from build123d import *

# Parameters (mm, degrees)
SKETCH1_W                           = 96.1517
SKETCH1_H                           = 78.74
BASE_PLATE_DEPTH                    = 2
SKETCH2_W                           = 5.08
SKETCH2_H                           = 5.08
SERVO_SUPPORTS_DEPTH                = 27.94
SKETCH3_R                           = 0.635
SERVO_MOUNT_HOLES_DEPTH             = 12.7
STRAP_HOLES_REACH                   = 70.132
SERVO_MOUNT_SPACING_COUNT           = 2
SERVO_MOUNT_SPACING_PITCH           = 38.1
SERVO_MOUNT_SPACING_COPY_1_SKETCH_W = 5.08
SERVO_MOUNT_SPACING_COPY_1_SKETCH_H = 5.08
SERVO_MOUNT_SPACING_COPY_1_DEPTH    = 27.94
SERVO_MOUNT_SPACING_COPY_2_SKETCH_R = 0.635
SERVO_MOUNT_SPACING_COPY_2_DEPTH    = 12.7
SKETCH11_W                          = 2.54
SKETCH11_H                          = 39.37
RACK_RAILS_DEPTH                    = 2.54


with BuildPart() as part:
    # Sketch1 → Base Plate (new body)
    with BuildSketch(Plane(origin=(0, 0, 0), x_dir=(1, 0, 0), z_dir=(0, 1, 0))):
        Rectangle(SKETCH1_W, SKETCH1_H)
    extrude(amount=BASE_PLATE_DEPTH)

    # Sketch2 → Servo Supports (add)
    with BuildSketch(Plane(origin=(0, 2, 0), x_dir=(1, 0, 0), z_dir=(0, 1, 0))):
        with Locations((20.13585, -30.48)):
            Rectangle(SKETCH2_W, SKETCH2_H)
        with Locations((20.13585, -2.54)):
            Rectangle(SKETCH2_W, SKETCH2_H)
    servo_supports = extrude(amount=SERVO_SUPPORTS_DEPTH)

    # Sketch3 → Servo Mount Holes (cut)
    with BuildSketch(Plane(origin=(22.67585, 0, 0), x_dir=(0, 0, -1), z_dir=(1, 0, 0))):
        with Locations((-30.504257117, 23.59)):
            Circle(SKETCH3_R)
        with Locations((-2.792857117, 23.59)):
            Circle(SKETCH3_R)
    servo_mount_holes = extrude(amount=-SERVO_MOUNT_HOLES_DEPTH, mode=Mode.SUBTRACT)

    # Sketch4 → Strap Holes (cut, up to next)
    with BuildSketch(Plane(origin=(0, 2, 0), x_dir=(1, 0, 0), z_dir=(0, 1, 0)), mode=Mode.PRIVATE) as strap_holes_sk1:
        with BuildLine():
            Line((45.53585, -24.17), (45.53585, -33.02))
            ThreePointArc((45.53585, -33.02), (44.53585, -34.02), (43.53585, -33.02))
            Line((43.53585, -33.02), (43.53585, -24.17))
            ThreePointArc((43.53585, -24.17), (44.53585, -23.17), (45.53585, -24.17))
        make_face()
    strap_holes_tool1 = extrude(strap_holes_sk1.sketch, amount=-STRAP_HOLES_REACH, mode=Mode.PRIVATE) & part.part
    # Sketch4 → Strap Holes (cut, up to next)
    with BuildSketch(Plane(origin=(0, 2, 0), x_dir=(1, 0, 0), z_dir=(0, 1, 0)), mode=Mode.PRIVATE) as strap_holes_sk2:
        with BuildLine():
            Line((45.53585, 33.02), (45.53585, 24.17))
            ThreePointArc((45.53585, 24.17), (44.53585, 23.17), (43.53585, 24.17))
            Line((43.53585, 24.17), (43.53585, 33.02))
            ThreePointArc((43.53585, 33.02), (44.53585, 34.02), (45.53585, 33.02))
        make_face()
    strap_holes_tool2 = extrude(strap_holes_sk2.sketch, amount=-STRAP_HOLES_REACH, mode=Mode.PRIVATE) & part.part
    # Sketch4 → Strap Holes (cut, up to next)
    with BuildSketch(Plane(origin=(0, 2, 0), x_dir=(1, 0, 0), z_dir=(0, 1, 0)), mode=Mode.PRIVATE) as strap_holes_sk3:
        with BuildLine():
            Line((-43.63085, -24.17), (-43.63085, -33.02))
            ThreePointArc((-43.63085, -33.02), (-44.63085, -34.02), (-45.63085, -33.02))
            Line((-45.63085, -33.02), (-45.63085, -24.17))
            ThreePointArc((-45.63085, -24.17), (-44.63085, -23.17), (-43.63085, -24.17))
        make_face()
    strap_holes_tool3 = extrude(strap_holes_sk3.sketch, amount=-STRAP_HOLES_REACH, mode=Mode.PRIVATE) & part.part
    # Sketch4 → Strap Holes (cut, up to next)
    with BuildSketch(Plane(origin=(0, 2, 0), x_dir=(1, 0, 0), z_dir=(0, 1, 0)), mode=Mode.PRIVATE) as strap_holes_sk4:
        with BuildLine():
            Line((-43.63085, 33.02), (-43.63085, 24.17))
            ThreePointArc((-43.63085, 24.17), (-44.63085, 23.17), (-45.63085, 24.17))
            Line((-45.63085, 24.17), (-45.63085, 33.02))
            ThreePointArc((-45.63085, 33.02), (-44.63085, 34.02), (-43.63085, 33.02))
        make_face()
    strap_holes_tool4 = extrude(strap_holes_sk4.sketch, amount=-STRAP_HOLES_REACH, mode=Mode.PRIVATE) & part.part
    # Sketch4 → Strap Holes (cut, up to next)
    with BuildSketch(Plane(origin=(0, 2, 0), x_dir=(1, 0, 0), z_dir=(0, 1, 0)), mode=Mode.PRIVATE) as strap_holes_sk5:
        with BuildLine():
            Line((45.53585, 4.425), (45.53585, -4.425))
            ThreePointArc((45.53585, -4.425), (44.53585, -5.425), (43.53585, -4.425))
            Line((43.53585, -4.425), (43.53585, 4.425))
            ThreePointArc((43.53585, 4.425), (44.53585, 5.425), (45.53585, 4.425))
        make_face()
    strap_holes_tool5 = extrude(strap_holes_sk5.sketch, amount=-STRAP_HOLES_REACH, mode=Mode.PRIVATE) & part.part
    # Sketch4 → Strap Holes (cut, up to next)
    with BuildSketch(Plane(origin=(0, 2, 0), x_dir=(1, 0, 0), z_dir=(0, 1, 0)), mode=Mode.PRIVATE) as strap_holes_sk6:
        with BuildLine():
            Line((-43.63085, 4.425), (-43.63085, -4.425))
            ThreePointArc((-43.63085, -4.425), (-44.63085, -5.425), (-45.63085, -4.425))
            Line((-45.63085, -4.425), (-45.63085, 4.425))
            ThreePointArc((-45.63085, 4.425), (-44.63085, 5.425), (-43.63085, 4.425))
        make_face()
    strap_holes_tool6 = extrude(strap_holes_sk6.sketch, amount=-STRAP_HOLES_REACH, mode=Mode.PRIVATE) & part.part
    # Sketch4 → Strap Holes (cut, up to next)
    with BuildSketch(Plane(origin=(0, 2, 0), x_dir=(1, 0, 0), z_dir=(0, 1, 0)), mode=Mode.PRIVATE) as strap_holes_sk7:
        with BuildLine():
            Line((41.72585, -24.17), (41.72585, -33.02))
            ThreePointArc((41.72585, -33.02), (40.72585, -34.02), (39.72585, -33.02))
            Line((39.72585, -33.02), (39.72585, -24.17))
            ThreePointArc((39.72585, -24.17), (40.72585, -23.17), (41.72585, -24.17))
        make_face()
    strap_holes_tool7 = extrude(strap_holes_sk7.sketch, amount=-STRAP_HOLES_REACH, mode=Mode.PRIVATE) & part.part
    # Sketch4 → Strap Holes (cut, up to next)
    with BuildSketch(Plane(origin=(0, 2, 0), x_dir=(1, 0, 0), z_dir=(0, 1, 0)), mode=Mode.PRIVATE) as strap_holes_sk8:
        with BuildLine():
            Line((41.72585, 33.02), (41.72585, 24.17))
            ThreePointArc((41.72585, 24.17), (40.72585, 23.17), (39.72585, 24.17))
            Line((39.72585, 24.17), (39.72585, 33.02))
            ThreePointArc((39.72585, 33.02), (40.72585, 34.02), (41.72585, 33.02))
        make_face()
    strap_holes_tool8 = extrude(strap_holes_sk8.sketch, amount=-STRAP_HOLES_REACH, mode=Mode.PRIVATE) & part.part
    # Sketch4 → Strap Holes (cut, up to next)
    with BuildSketch(Plane(origin=(0, 2, 0), x_dir=(1, 0, 0), z_dir=(0, 1, 0)), mode=Mode.PRIVATE) as strap_holes_sk9:
        with BuildLine():
            Line((41.72585, 4.425), (41.72585, -4.425))
            ThreePointArc((41.72585, -4.425), (40.72585, -5.425), (39.72585, -4.425))
            Line((39.72585, -4.425), (39.72585, 4.425))
            ThreePointArc((39.72585, 4.425), (40.72585, 5.425), (41.72585, 4.425))
        make_face()
    strap_holes_tool9 = extrude(strap_holes_sk9.sketch, amount=-STRAP_HOLES_REACH, mode=Mode.PRIVATE) & part.part
    # Sketch4 → Strap Holes (cut, up to next)
    with BuildSketch(Plane(origin=(0, 2, 0), x_dir=(1, 0, 0), z_dir=(0, 1, 0)), mode=Mode.PRIVATE) as strap_holes_sk10:
        with BuildLine():
            Line((-39.82085, -24.17), (-39.82085, -33.02))
            ThreePointArc((-39.82085, -33.02), (-40.82085, -34.02), (-41.82085, -33.02))
            Line((-41.82085, -33.02), (-41.82085, -24.17))
            ThreePointArc((-41.82085, -24.17), (-40.82085, -23.17), (-39.82085, -24.17))
        make_face()
    strap_holes_tool10 = extrude(strap_holes_sk10.sketch, amount=-STRAP_HOLES_REACH, mode=Mode.PRIVATE) & part.part
    # Sketch4 → Strap Holes (cut, up to next)
    with BuildSketch(Plane(origin=(0, 2, 0), x_dir=(1, 0, 0), z_dir=(0, 1, 0)), mode=Mode.PRIVATE) as strap_holes_sk11:
        with BuildLine():
            Line((-39.82085, 33.02), (-39.82085, 24.17))
            ThreePointArc((-39.82085, 24.17), (-40.82085, 23.17), (-41.82085, 24.17))
            Line((-41.82085, 24.17), (-41.82085, 33.02))
            ThreePointArc((-41.82085, 33.02), (-40.82085, 34.02), (-39.82085, 33.02))
        make_face()
    strap_holes_tool11 = extrude(strap_holes_sk11.sketch, amount=-STRAP_HOLES_REACH, mode=Mode.PRIVATE) & part.part
    # Sketch4 → Strap Holes (cut, up to next)
    with BuildSketch(Plane(origin=(0, 2, 0), x_dir=(1, 0, 0), z_dir=(0, 1, 0)), mode=Mode.PRIVATE) as strap_holes_sk12:
        with BuildLine():
            Line((-39.82085, 4.425), (-39.82085, -4.425))
            ThreePointArc((-39.82085, -4.425), (-40.82085, -5.425), (-41.82085, -4.425))
            Line((-41.82085, -4.425), (-41.82085, 4.425))
            ThreePointArc((-41.82085, 4.425), (-40.82085, 5.425), (-39.82085, 4.425))
        make_face()
    strap_holes_tool12 = extrude(strap_holes_sk12.sketch, amount=-STRAP_HOLES_REACH, mode=Mode.PRIVATE) & part.part
    add(strap_holes_tool1.solids().sort_by_distance((44.53585, 2, 28.595))[0], mode=Mode.SUBTRACT)
    add(strap_holes_tool2.solids().sort_by_distance((44.53585, 2, -28.595))[0], mode=Mode.SUBTRACT)
    add(strap_holes_tool3.solids().sort_by_distance((-44.63085, 2, 28.595))[0], mode=Mode.SUBTRACT)
    add(strap_holes_tool4.solids().sort_by_distance((-44.63085, 2, -28.595))[0], mode=Mode.SUBTRACT)
    add(strap_holes_tool5.solids().sort_by_distance((44.53585, 2, 0))[0], mode=Mode.SUBTRACT)
    add(strap_holes_tool6.solids().sort_by_distance((-44.63085, 2, 0))[0], mode=Mode.SUBTRACT)
    add(strap_holes_tool7.solids().sort_by_distance((40.72585, 2, 28.595))[0], mode=Mode.SUBTRACT)
    add(strap_holes_tool8.solids().sort_by_distance((40.72585, 2, -28.595))[0], mode=Mode.SUBTRACT)
    add(strap_holes_tool9.solids().sort_by_distance((40.72585, 2, 0))[0], mode=Mode.SUBTRACT)
    add(strap_holes_tool10.solids().sort_by_distance((-40.82085, 2, 28.595))[0], mode=Mode.SUBTRACT)
    add(strap_holes_tool11.solids().sort_by_distance((-40.82085, 2, -28.595))[0], mode=Mode.SUBTRACT)
    add(strap_holes_tool12.solids().sort_by_distance((-40.82085, 2, 0))[0], mode=Mode.SUBTRACT)

    # Servo Mount Mirror: Servo Supports, Servo Mount Holes across plane
    add(servo_supports.mirror(Plane(origin=(0, 0, 0), x_dir=(0, 0, 1), z_dir=(1, 0, 0))))
    add(servo_mount_holes.mirror(Plane(origin=(0, 0, 0), x_dir=(0, 0, 1), z_dir=(1, 0, 0))), mode=Mode.SUBTRACT)

    # Servo Mount Spacing: Servo Supports, Servo Mount Holes ×2
    with Locations(*[(0, 0, -i * SERVO_MOUNT_SPACING_PITCH) for i in range(1, SERVO_MOUNT_SPACING_COUNT)]):
        add(servo_supports)
        add(servo_mount_holes, mode=Mode.SUBTRACT)

    # Servo Mount Spacing copy 1 sketch → Servo Mount Spacing copy 1 (add)
    with BuildSketch(Plane(origin=(0, 2, -38.1), x_dir=(-1, 0, 0), z_dir=(0, 1, 0))):
        with Locations((20.13585, 30.48)):
            Rectangle(SERVO_MOUNT_SPACING_COPY_1_SKETCH_W, SERVO_MOUNT_SPACING_COPY_1_SKETCH_H)
        with Locations((20.13585, 2.54)):
            Rectangle(SERVO_MOUNT_SPACING_COPY_1_SKETCH_W, SERVO_MOUNT_SPACING_COPY_1_SKETCH_H)
    extrude(amount=SERVO_MOUNT_SPACING_COPY_1_DEPTH)

    # Servo Mount Spacing copy 2 sketch → Servo Mount Spacing copy 2 (cut)
    with BuildSketch(Plane(origin=(-22.67585, 0, -38.1), x_dir=(0, 0, -1), z_dir=(-1, 0, 0))):
        with Locations((-30.504257117, -23.59)):
            Circle(SERVO_MOUNT_SPACING_COPY_2_SKETCH_R)
        with Locations((-2.792857117, -23.59)):
            Circle(SERVO_MOUNT_SPACING_COPY_2_SKETCH_R)
    extrude(amount=-SERVO_MOUNT_SPACING_COPY_2_DEPTH, mode=Mode.SUBTRACT)

    # Sketch11 → Rack Rails (add)
    with BuildSketch(Plane(origin=(0, 2, 0), x_dir=(1, 0, 0), z_dir=(0, 1, 0))):
        with Locations((31.56585, -19.685)):
            Rectangle(SKETCH11_W, SKETCH11_H)
        with Locations((37.78885, -19.685)):
            Rectangle(SKETCH11_W, SKETCH11_H)
    extrude(amount=RACK_RAILS_DEPTH)


solid = part.part
Design review of the part built by this model. Coordinates are the model's own, in mm. A direction names the side the tool comes from. Give positions to 0.01 mm unless a question says otherwise; leave off trailing zeros. Loops run counter-clockwise (first coordinate to the right, second up) from the corner with the lowest first, then second, coordinate; pieces in that order, holes last. Notation, with made-up numbers: M 66.25,37 L 86.25,37 A25 cw 86.25,58 Z; hole C 70,30 d6. An arc over 180 degrees is marked long. One line per question, with ' | ' between items. Start each with the question number.
1. Add section B-B (x = 21). Write out the cut boundary in (y, z) (3 decimals), plus the area to 3 significant figures.
2. For faces 4 (the face through (-20, 16, -38.1)), 5 (the face through (22.676, 16, -36)), 6 (the face through (-20, 16, -5.08)), 7 (the face through (-22.676, 16, -8)), 8 (the face through (45.536, 1, -29)), list the 3-axis set-ups (+Z, -Z, +X, -X, +Y, -Y) from which the entire face can be reached by the end or side of a thin tool; tool diameter is ignored.
3. The part is to be moulded in two halves that separate along Z. For faces 1 (the face through (-20, 16, -33.02)), 2 (the face through (20, 16, 33.02)), 3 (the face through (17.596, 16, -36)), say which applies: released by +Z, released by -Z, zero draft, split by the parting line, or undercut.
4. Add section A-A (y = 16). Give the number of separate pieces and of enclosed holes in the cut face, plus the area to 3 significant figures.
5. Add section D-D (x = 9.5). Write out the cut boundary in (y, z).
6. Add section C-C (z = -21.5). Write out the cut boundary in (x, y).
7. Insertion check: P1, Ø12, axis at x = 17.5, z = -26.5, coming from the +Y side; P2, Ø1.5, axis at y = 16, z = -36, coming from the -X side; P3, Ø1.5, axis at x = 21, y = 21, coming from the -Z side. Each pin has a flat end and moves straight along its axis. Give the tip position at first contact, or say it passes through.
8. To check wall thickness, follow L1, parallel to Z at x = -20.5, y = 4; L2, parallel to X at y = 17.5, z = 29; L3, parallel to Y at x = -5, z = -33.5. State the ranges of each line that lie inside material, in increasing order.
Worked out:
1) outline: M 0,-39.37 L 2,-39.37 L 2,-38.1 L 29.94,-38.1 L 29.94,-33.02 L 2,-33.02 L 2,-10.16 L 29.94,-10.16 L 29.94,-5.08 L 2,-5.08 L 2,0 L 29.94,0 L 29.94,5.08 L 2,5.08 L 2,27.94 L 29.94,27.94 L 29.94,33.02 L 2,33.02 L 2,39.37 L 0,39.37 Z; hole C 23.59,-35.307 d1.27; hole C 23.59,-7.596 d1.27; hole C 23.59,2.793 d1.27; hole C 23.59,30.504 d1.27 | area: 720 mm²
2) face 4: -Z, +X, -X, +Y | face 5: +Z, -Z, +X, +Y | face 6: +X, -X, +Y | face 7: +Z, -Z, -X, +Y | face 8: +Y, -Y
3) face 1: undercut | face 2: released by +Z | face 3: zero draft
4) separate pieces: 8 | enclosed holes: 0 | area: 206 mm²
5) outline: M 0,-39.37 L 2,-39.37 L 2,39.37 L 0,39.37 Z
6) outline: M -48.08,0 L 48.08,0 L 48.08,2 L -48.08,2 Z
7) P1: stops at y = 2 | P2: stops at x = -22.68 | P3: stops at z = -38.1
8) L1: z = -38.1 to -33.02, -10.16 to -5.08, 0 to 5.08, 27.94 to 33.02 | L2: x = -22.68 to -17.6, 17.6 to 22.68 | L3: y = 0 to 2
